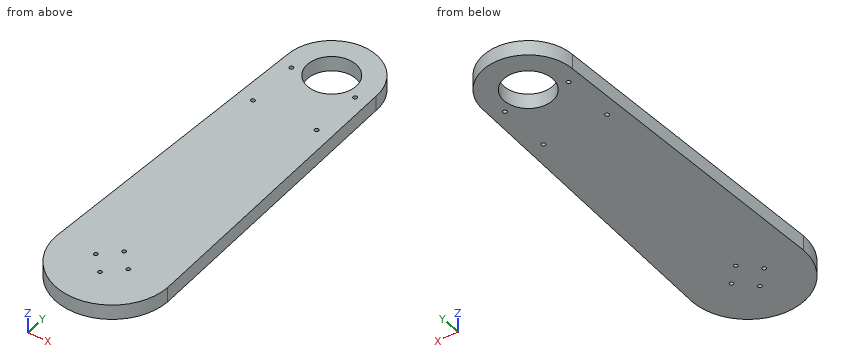
from build123d import *

# Parameters (mm, degrees)
BOSS_EXTRUDE1_DEPTH = 10
CUT_EXTRUDE4_REACH  = 12
SKETCH3_R           = 16.25
CUT_EXTRUDE5_REACH  = 12
SKETCH4_R           = 1.3
SKETCH5_R           = 1.35
CUT_EXTRUDE6_DEPTH  = 10


with BuildPart() as part:
    # Sketch1 → Boss-Extrude1 (new body)
    with BuildSketch(Plane.XY):
        with BuildLine():
            ThreePointArc((30, 200), (0, 230), (-30, 200))
            Line((-30, 200), (-37.5, 0))
            ThreePointArc((-37.5, 0), (0, -37.5), (37.5, 0))
            Line((37.5, 0), (30, 200))
        make_face()
    extrude(amount=BOSS_EXTRUDE1_DEPTH)

    # Sketch3 → Cut-Extrude4 (cut, up to next)
    with BuildSketch(Plane(origin=(0, 0, 0), x_dir=(-1, 0, 0), z_dir=(0, 0, -1)), mode=Mode.PRIVATE) as cut_extrude4_sk1:
        with Locations((0, 200)):
            Circle(SKETCH3_R)
    cut_extrude4_tool1 = extrude(cut_extrude4_sk1.sketch, amount=-CUT_EXTRUDE4_REACH, mode=Mode.PRIVATE) & part.part
    add(cut_extrude4_tool1.solids().sort_by_distance((0, 200, 0))[0], mode=Mode.SUBTRACT)

    # Sketch4 → Cut-Extrude5 (cut, up to next)
    with BuildSketch(Plane(origin=(0, 0, 0), x_dir=(-1, 0, 0), z_dir=(0, 0, -1)), mode=Mode.PRIVATE) as cut_extrude5_sk1:
        with Locations((0, 11)):
            Circle(SKETCH4_R)
    cut_extrude5_tool1 = extrude(cut_extrude5_sk1.sketch, amount=-CUT_EXTRUDE5_REACH, mode=Mode.PRIVATE) & part.part
    add(cut_extrude5_tool1.solids().sort_by_distance((0, 11, 0))[0], mode=Mode.SUBTRACT)
    # Sketch4 → Cut-Extrude5 (cut, up to next)
    with BuildSketch(Plane(origin=(0, 0, 0), x_dir=(-1, 0, 0), z_dir=(0, 0, -1)), mode=Mode.PRIVATE) as cut_extrude5_sk2:
        with Locations((11, 0)):
            Circle(SKETCH4_R)
    cut_extrude5_tool2 = extrude(cut_extrude5_sk2.sketch, amount=-CUT_EXTRUDE5_REACH, mode=Mode.PRIVATE) & part.part
    add(cut_extrude5_tool2.solids().sort_by_distance((-11, 0, 0))[0], mode=Mode.SUBTRACT)
    # Sketch4 → Cut-Extrude5 (cut, up to next)
    with BuildSketch(Plane(origin=(0, 0, 0), x_dir=(-1, 0, 0), z_dir=(0, 0, -1)), mode=Mode.PRIVATE) as cut_extrude5_sk3:
        with Locations((0, -11)):
            Circle(SKETCH4_R)
    cut_extrude5_tool3 = extrude(cut_extrude5_sk3.sketch, amount=-CUT_EXTRUDE5_REACH, mode=Mode.PRIVATE) & part.part
    add(cut_extrude5_tool3.solids().sort_by_distance((0, -11, 0))[0], mode=Mode.SUBTRACT)
    # Sketch4 → Cut-Extrude5 (cut, up to next)
    with BuildSketch(Plane(origin=(0, 0, 0), x_dir=(-1, 0, 0), z_dir=(0, 0, -1)), mode=Mode.PRIVATE) as cut_extrude5_sk4:
        with Locations((-11, 0)):
            Circle(SKETCH4_R)
    cut_extrude5_tool4 = extrude(cut_extrude5_sk4.sketch, amount=-CUT_EXTRUDE5_REACH, mode=Mode.PRIVATE) & part.part
    add(cut_extrude5_tool4.solids().sort_by_distance((11, 0, 0))[0], mode=Mode.SUBTRACT)

    # Sketch5 → Cut-Extrude6 (cut)
    with BuildSketch(Plane(origin=(0, 0, 0), x_dir=(-1, 0, 0), z_dir=(0, 0, -1))):
        with Locations((21.5, 157.25)):
            Circle(SKETCH5_R)
        with Locations((-21.5, 157.25)):
            Circle(SKETCH5_R)
        with Locations((-21.5, 192.25)):
            Circle(SKETCH5_R)
        with Locations((21.5, 192.25)):
            Circle(SKETCH5_R)
    extrude(amount=-CUT_EXTRUDE6_DEPTH, mode=Mode.SUBTRACT)


solid = part.part
Source: CAD feature listing. Evaluate the final solid. Frame: model axes, mm. Give positions to 0.01 mm unless a question says otherwise; leave off trailing zeros. Order: outer loops, then holes, each group sorted by start corner. A loop starts at its lowest first (then second) coordinate and runs counter-clockwise, first axis right, second up. Notation, with made-up numbers: (-17.5, 81.5) -> (-3.5, 81.5) arc R24 cw to (-3.5, 104.5) -> close; hole circle Ø1 at (74, -38). An arc over 180 degrees is marked (long way). Use a Markdown table: item, result.
1) Section query C-C, the plane y = 197. Return the cut outline in (x, z).
Answer list:
| item | result |
|---|---|
| outline | (-30.11, 0) -> (-15.97, 0) -> (-15.97, 10) -> (-30.11, 10) -> close; (15.97, 0) -> (30.11, 0) -> (30.11, 10) -> (15.97, 10) -> close |
2) Section query B-B, the plane x = -4. Return the cut outline in (y, z), then the cut area to 3 significant figures.
Answer list:
| item | result |
|---|---|
| outline | (-37.29, 0) -> (184.25, 0) -> (184.25, 10) -> (-37.29, 10) -> close; (215.75, 0) -> (229.73, 0) -> (229.73, 10) -> (215.75, 10) -> close |
| area | 2,360 mm² |
3) Section query A-A, the plane z = 6. Count the separate pieces of the cut face and the enclosed holes in it, then the cut area to 3 significant figures.
Answer list:
| item | result |
|---|---|
| separate pieces | 1 |
| enclosed holes | 9 |
| area | 16,200 mm² |
4) Contact query for flat-ended pins moving along their axis: P1, Ø4, axis at y = 144, z = 5.5, coming from the -X side (3 decimals); P2, Ø1, axis at y = 124.5, z = 8, coming from the +X side; P3, Ø1.6, axis at x = 0, y = -11, coming from the -Z side; P4, Ø5, axis at y = 203, z = 5, coming from the +X side. Output: stop coordinate, or through.
Answer list:
| item | result |
|---|---|
| P1 | x = -32.175 |
| P2 | x = 32.85 |
| P3 | through |
| P4 | x = 30 |
5) Section query D-D, the plane y = 132. Return the cut outline in (x, z), then the cut area to 3 significant figures.
Answer list:
| item | result |
|---|---|
| outline | (-32.55, 0) -> (32.55, 0) -> (32.55, 10) -> (-32.55, 10) -> close |
| area | 651 mm² |
6) Ray query, line 1 along Y through (x, z) = (0, 7.75); line 2 along Y through (x, z) = (-12, 3.5); line 3 along Y through (x, z) = (21, 8.25). Return the intervals inside material, ascending. Write a range as [from, to].
Answer list:
| item | result |
|---|---|
| line 1 | [-37.5, -12.3], [-9.7, 9.7], [12.3, 183.75], [216.25, 230] |
| line 2 | [-35.53, -0.83], [0.83, 189.04], [210.96, 227.5] |
| line 3 | [-31.07, 156], [158.5, 191], [193.5, 221.42] |
